Solid Edge part; units mm, degrees
sketch "Sketch1" plane through (0, 0, 0) normal (0, 0, 1) x (1, 0, 0)
  circle A0 centre (0, 0) radius 4.25
extrude "Protrusion1" add sketch "Sketch1" along normal blind 5
sketch "Sketch2" plane through (0, 0, 5) normal (0, 0, 1) x (1, 0, 0)
  circle A0 centre (0, 0) radius 2.5
extrude "ExtrudedProtrusion_2" add sketch "Sketch2" along normal blind 50
sketch "Sketch3" plane through (0, 0, 0) normal (0, 0, -1) x (-1, 0, 0)
  line L0 (2.25, 0) -> (1.125, 1.9486)
  line L1 (1.125, 1.9486) -> (-1.125, 1.9486)
  line L2 (-1.125, 1.9486) -> (-2.25, 0)
  line L3 (-2.25, 0) -> (-1.125, -1.9486)
  line L4 (-1.125, -1.9486) -> (1.125, -1.9486)
  line L5 (1.125, -1.9486) -> (2.25, 0)
extrude "ExtrudedCutout_1" cut sketch "Sketch3" against normal blind 2.6
cosmetic_thread "Thread_1" thread depth 24
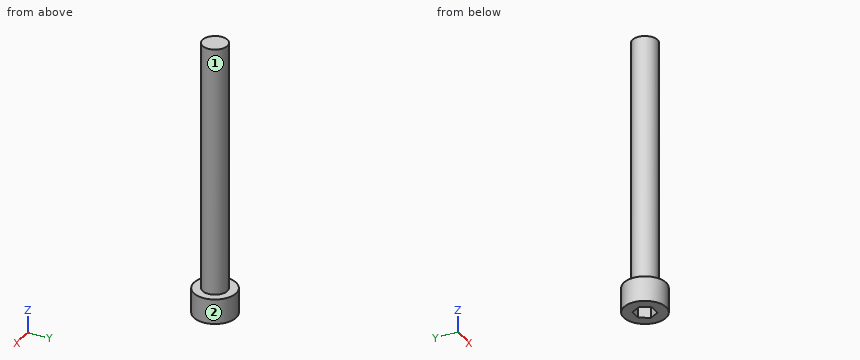
Build history of the part. All positions in model axes, mm. Face numbers are marked on the shaded views. A direction names the side the tool comes from. Coordinates: 2 decimals unless noted, no trailing zeros. Write each loop counter-clockwise with the first axis right and the second up, starting at its lowest first coordinate (ties: lowest second). Pieces come first, ordered by that corner, then holes.
1. Drop flat-ended pins along their axis: pin 1 (4 mm diameter, centred on x = -1, y = -3, fed in from +Z); pin 2 (0.7 mm diameter, centred on x = -0.5, z = 1, fed in from +Y); pin 3 (4 mm diameter, centred on x = 2, z = 34.5, fed in from -Y). Give the stop position or say it passes through.
Answer block:
pin 1: stops at z = 55
pin 2: stops at y = 4.25
pin 3: stops at y = -2.5
2. Band-saw the part on C-C, the plane y = -3. Give the cut face in (x, z), and give its area (3 significant figures).
Answer block:
outline: (-3.01, 0) - (3.01, 0) - (3.01, 5) - (-3.01, 5) - close
area: 30.1 mm2
3. 3-axis set-ups, long thin cutter, end or side, ignore diameter. For the marked faces 1 and 2: which of +Z, -Z, +X, -X, +Y, -Y reach the whole face in a straight line?
Answer block:
face 1: +Z
face 2: +Z, -Z
4. Band-saw the part on A-A, the plane x = 0. Give the cut face in (y, z).
Answer block:
outline: (-4.25, 0) - (-1.95, 0) - (-1.95, 2.6) - (1.95, 2.6) - (1.95, 0) - (4.25, 0) - (4.25, 5) - (2.5, 5) - (2.5, 55) - (-2.5, 55) - (-2.5, 5) - (-4.25, 5) - close
5. Drill centre lines: probe 1 along Z at (x, y) = (-2, -1.75); probe 2 along Y at (x, z) = (0, 35.5); probe 3 along Z at (x, y) = (-0.75, 1.5). Where is each one in solid material? Low to high.
Answer block:
probe 1: z = 0 to 5
probe 2: y = -2.5 to 2.5
probe 3: z = 2.6 to 55
6. Band-saw the part on B-B, the plane z = 38. Give the cut face in (x, y), and give its area (3 significant figures).
Answer block:
outline: circle Ø5 at (0, 0)
area: 19.6 mm2
